Part model, mm, in its own coordinate system. A direction names the side the tool comes from. Give positions to 0.01 mm unless a question says otherwise; leave off trailing zeros. Write each loop counter-clockwise with the first axis right and the second up, starting at its lowest first coordinate (ties: lowest second). Pieces come first, ordered by that corner, then holes. Notation, with made-up numbers: M -7,-3.5 L 30,-3.5 A7 cw 30,3.5 Z; hole C 22.5,15 d5. An arc over 180 degrees is marked long. Use CSV: the item, a comma, the result in double quotes. Start each with the question number.
1. 3-axis set-ups, long thin cutter, end or side, ignore diameter. For faces 4 (the face through (-39.39, 21.48, 23.98)), 5 (the face through (-35, 20, 18)), 6 (the face through (-35.1, 23.16, 6.69)): which of +Z, -Z, +X, -X, +Y, -Y reach the whole face in a straight line?
2. Band-saw the part on A-A, the plane z = 7. List the corners of the cut face in (x, y), then the cut area to 3 significant figures.
3. Band-saw the part on D-D, the plane z = 23. List the corners of the cut face in (x, y).
4. Drill centre lines: line 1 along X through (y, z) = (15.3, 5.25); line 2 along Z through (x, y) = (-36.25, 25); line 3 along Y through (x, z) = (-38, 17). Where is each one in solid material? Low to high. Write a range as from..to.
5. Band-saw the part on B-B, the plane y = 25. List the corners of the cut face in (x, z).
6. Mould opens along Z. For faces 1 (the face through (-35, 23, 23)), 2 (the face through (-33.31, 17.14, 5.07)), 3 (the face through (-41.14, 25.07, 29.1)) say: pulls with the +Z half, pulls with the -Z half, needs draft (parallel to the pull), parting line crosses it, or undercut.
7. Band-saw the part on C-C, the plane x = -37. List the corners of the cut face in (y, z).
8. Drop flat-ended pins along their axis: pin 1 Ø1.5 at (x, z) = (-31.5, 19) entering from -Y; pin 2 Ø4 at (x, y) = (-38.5, 16) entering from +Z; pin 3 Ø4.5 at (y, z) = (25, 5) entering from +X; pin 4 Ø2.5 at (x, z) = (-34, 23.5) entering from -Y. Give the stop position or say it passes through.
from build123d import *

# Parameters (mm, degrees)
SKETCH002_R     = 2.5
PAD001_DEPTH    = 7
SKETCH003_R     = 4.5
POCKET001_DEPTH = 3
FILLET_R        = 3
SKETCH004_R     = 2.5
POCKET002_DEPTH = 10.001
FILLET001_R     = 1


with BuildPart() as part:
    # Sketch002 → Pad001 (new body, symmetric)
    with BuildSketch(Plane.YZ):
        Polygon((10, 10), (20, 10), (20, 30), (30, 30), (30, 0), (5, 0), align=None)
        with Locations((25, 5)):
            Circle(SKETCH002_R, mode=Mode.SUBTRACT)
    extrude(amount=PAD001_DEPTH, both=True)

    # Sketch003 (on Face2 of Pad001) → Pocket001 (cut)
    with BuildSketch(Plane(origin=(0, 20, 0), x_dir=(0, 0, -1), z_dir=(0, -1, 0))):
        with Locations((-23, 0)):
            Circle(SKETCH003_R)
    extrude(amount=-POCKET001_DEPTH, mode=Mode.SUBTRACT)

    # Fillet
    fillet_edges = [part.edges().sort_by_distance(p)[0] for p in [
        (-7, 25, 30),
        (7, 25, 30),
    ]]
    fillet(fillet_edges, radius=FILLET_R)

    # Sketch004 (on Face4 of Fillet) → Pocket002 (cut, through all)
    with BuildSketch(Plane(origin=(0, 0, 10), x_dir=(0, -1, 0), z_dir=(0, 0, 1))):
        with Locations((-15.3, 0)):
            Circle(SKETCH004_R)
    extrude(amount=-POCKET002_DEPTH, mode=Mode.SUBTRACT)

    # Fillet001
    fillet001_edges = [part.edges().sort_by_distance(p)[0] for p in [
        (0, 20, 10),
    ]]
    fillet(fillet001_edges, radius=FILLET001_R)


with BuildPart() as part_1:
    # Body001 placement: moved
    add(part.part.moved(Location((-35, 0, 0))))


solid = part_1.part
Output:
1,face 4,"-Y"
1,face 5,"+Z, +X, -X, -Y"
1,face 6,"+X, -X"
2,outline,"M -42,8.5 L -28,8.5 L -28,23.5 L -42,23.5 Z; M -42,26.5 L -28,26.5 L -28,30 L -42,30 Z; hole C -35,15.3 d5"
2,area,"239 mm²"
3,outline,"M -42,20 L -39.5,20 L -39.5,23 L -30.5,23 L -30.5,20 L -28,20 L -28,30 L -42,30 Z"
4,line 1,"x = -42..-37.5, -32.5..-28"
4,line 2,"z = 0..2.5, 7.5..30"
4,line 3,"y = 20..30"
5,outline,"M -42,0 L -28,0 L -28,2.5 L -42,2.5 Z; M -42,7.5 L -28,7.5 L -28,27 A3 ccw -31,30 L -39,30 A3 ccw -42,27 Z"
6,face 1,"undercut"
6,face 2,"needs draft"
6,face 3,"pulls with the +Z half"
7,outline,"M 5,0 L 13.8,0 L 13.8,10 L 10,10 Z; M 16.8,0 L 30,0 L 30,30 L 20,30 L 20,27.03 L 23,27.03 L 23,18.97 L 20,18.97 L 20,11 A1 cw 19,10 L 16.8,10 Z; hole C 25,5 d5"
8,pin 1,"stops at y = 20"
8,pin 2,"stops at z = 10"
8,pin 3,"passes through"
8,pin 4,"stops at y = 23"
